Could you check a few things on this model? Use its own coordinates, in mm. Face numbers are marked on the shaded views. A direction names the side the tool comes from. Give positions to 0.01 mm unless a question says otherwise; leave off trailing zeros. Write each loop counter-clockwise with the first axis right and the second up, starting at its lowest first coordinate (ties: lowest second). Pieces come first, ordered by that corner, then holes. Notation, with made-up numbers: (69, 72) - (76, 72) arc R18 ccw to (76, 82) - close; hole circle Ø7 at (10.5, 21). An arc over 180 degrees is marked (long way). Write item = value, one per line.
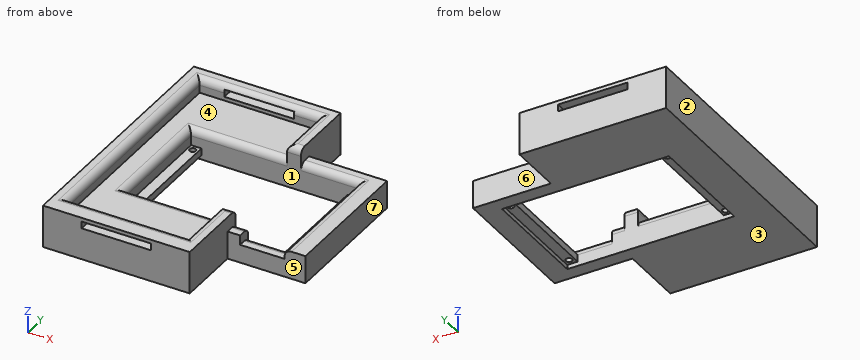
from build123d import *

# Parameters (mm, degrees)
F0_W      = 76.2
F0_H      = 50.8
F1_DEPTH  = 20.32
F2_W      = 60.96
F2_H      = 40.64
F3_DEPTH  = 17.272
F5_W      = 3.81
F5_H      = 40.64
F5_R      = 1.13665
F6_DEPTH  = 2.54
F8_W      = 16.256
F8_H      = 5.08
F9_DEPTH  = 3.4925
F11_DEPTH = 5.334
F13_DEPTH = 20.32
F14_R     = 2.54
F15_W     = 93.98
F15_H     = 10.16
F16_DEPTH = 82.042
F17_W     = 25.4
F17_H     = 2.54
F18_DEPTH = 93.98


with BuildPart() as f1:
    # F0 (on Top) → F1 (new body)
    with BuildSketch(Plane.XY):
        Rectangle(F0_W, F0_H)
    extrude(amount=F1_DEPTH)

    # F2 (on face) → F3 (cut)
    with BuildSketch(Plane.XY.offset(20.32)):
        Rectangle(F2_W, F2_H)
    extrude(amount=-F3_DEPTH, mode=Mode.SUBTRACT)

    # F5 (on offset) → F6 (join)
    with BuildSketch(Plane.XY.offset(11.7475)):
        with Locations((-28.575, 0)):
            Rectangle(F5_W, F5_H)
        with Locations((-28.575, -18.1356)):
            Circle(F5_R, mode=Mode.SUBTRACT)
        with Locations((-28.575, 18.1356)):
            Circle(F5_R, mode=Mode.SUBTRACT)
        with Locations((28.575, 0)):
            Rectangle(F5_W, F5_H)
        with Locations((28.575, -18.1356)):
            Circle(F5_R, mode=Mode.SUBTRACT)
        with Locations((28.575, 18.1356)):
            Circle(F5_R, mode=Mode.SUBTRACT)
    extrude(amount=F6_DEPTH)

    # F8 (on offset) → F9 (cut, through all)
    with BuildSketch(Plane.XY.offset(16.8275)):
        with Locations((22.352, -22.86)):
            Rectangle(F8_W, F8_H)
    extrude(amount=F9_DEPTH, mode=Mode.SUBTRACT)

    # F10 (on face) → F11 (join)
    with BuildSketch(Plane.XY.offset(20.32)):
        Polygon((-38.862, -41.3258), (-38.862, 39.9542), (4.572, 39.9542), (4.572, 20.32), (9.652, 20.32), (9.652, 45.0342), (-43.942, 45.0342), (-43.942, -48.9458), (9.652, -48.9458), (9.652, -20.32), (4.572, -20.32), (4.572, -41.3258), align=None)
    extrude(amount=F11_DEPTH)

    # F12 (on face) → F13 (join, through all)
    with BuildSketch(Plane(origin=(0, 0, 0), x_dir=(1, 0, 0), z_dir=(0, 0, -1))):
        Polygon((-43.942, 48.9458), (-43.942, -45.0342), (9.652, -45.0342), (9.652, -25.4), (-38.1, -25.4), (-38.1, 25.4), (9.652, 25.4), (9.652, 48.9458), align=None)
    extrude(amount=-F13_DEPTH)

    # F14
    f14_edges = [f1.edges().sort_by_distance(p)[0] for p in [
        (-12.954, 20.32, 20.32),
        (-30.48, 0, 20.32),
        (30.48, -2.54, 20.32),
        (-17.145, 39.9542, 25.654),
        (-38.862, -0.6858, 25.654),
        (-17.145, -41.3258, 25.654),
        (4.572, -30.8229, 25.654),
        (4.572, 30.1371, 25.654),
        (22.352, -20.32, 16.8275),
        (11.938, -20.32, 20.32),
        (-12.954, -20.32, 20.32),
        (20.066, 20.32, 20.32),
        (7.112, 20.32, 25.654),
        (7.112, -20.32, 25.654),
    ]]
    fillet(f14_edges, radius=F14_R)

    # F15 (on face) → F16 (cut, through all)
    with BuildSketch(Plane.YZ.offset(38.1)):
        with Locations((-1.9558, 5.08)):
            Rectangle(F15_W, F15_H)
    extrude(amount=-F16_DEPTH, mode=Mode.SUBTRACT)

    # F17 (on face) → F18 (cut, through all)
    with BuildSketch(Plane.XZ.offset(48.9458)):
        with Locations((-17.145, 22.987)):
            Rectangle(F17_W, F17_H)
    extrude(amount=-F18_DEPTH, mode=Mode.SUBTRACT)


solid = f1.part
1. Thinking about a two-plate mould opening in X: for the marked faces 1, 2, 3 and 4, which applies, pulls with the +X half, pulls with the -X half, needs draft (parallel to the pull), parting line crosses it, or undercut?
Filled sheet:
face_1 = undercut
face_2 = pulls with the -X half
face_3 = needs draft
face_4 = undercut
2. If we section it at C-C, the plane y = -37: Please give me the cut outline in (x, z), and give its area (3 significant figures).
Filled sheet:
outline = (-43.94, 10.16) - (9.65, 10.16) - (9.65, 25.65) - (7.11, 25.65) arc R2.54 ccw to (4.57, 23.11) - (4.57, 20.32) - (-38.86, 20.32) - (-38.86, 23.11) arc R2.54 ccw to (-41.4, 25.65) - (-43.94, 25.65) - close
area = 596 mm2
3. I need wall thicknesses on line 1 (X direction, y = -25, z = 21.75); line 2 (Y direction, x = -14, z = 12.25); line 3 (Y direction, x = -12.5, z = 21). Which ranges of each line are inside material? Lowest first, please.
Filled sheet:
line_1 = -43.94 to -38.86, 4.57 to 9.65
line_2 = -48.95 to -20.32, 20.32 to 45.03
line_3 = -48.95 to -41.33, 39.95 to 45.03
4. For pin 1 (2.5 mm diameter, centred on x = 28.58, y = 18.14, fed in from -Z); pin 2 (12 mm diameter, centred on x = -3.5, y = -30, fed in from +Z); pin 3 (0.8 mm diameter, centred on x = -24.5, z = 22, fed in from +Y); pin 4 (8 mm diameter, centred on x = 24.5, z = 13.5, fed in from +Y), each with a flat end and sliding along its axis, tell me the tip position at first contact or that it passes through.
Filled sheet:
pin_1 = 11.75
pin_2 = 20.32
pin_3 = 45.03
pin_4 = 25.4
5. If we section it at D-D, the plane x = -28.5: Count the separate pieces of the cut face and the enclosed holes in it, and give its area (3 significant figures).
Filled sheet:
separate_pieces = 5
enclosed_holes = 0
area = 664 mm2
6. If we section it at B-B, the plane y = -8: Please give me the cut outline in (x, z), and give its area (3 significant figures).
Filled sheet:
outline = (-43.94, 10.16) - (-30.48, 10.16) - (-30.48, 11.75) - (-26.67, 11.75) - (-26.67, 14.29) - (-30.48, 14.29) - (-30.48, 17.78) arc R2.54 ccw to (-33.02, 20.32) - (-38.86, 20.32) - (-38.86, 23.11) arc R2.54 ccw to (-41.4, 25.65) - (-43.94, 25.65) - close; (26.67, 11.75) - (30.48, 11.75) - (30.48, 10.16) - (38.1, 10.16) - (38.1, 20.32) - (33.02, 20.32) arc R2.54 ccw to (30.48, 17.78) - (30.48, 14.29) - (26.67, 14.29) - close
area = 256 mm2
7. If we section it at A-A, the plane x = -11: Please give me the cut outline in (y, z).
Filled sheet:
outline = (-48.95, 10.16) - (-20.32, 10.16) - (-20.32, 17.78) arc R2.54 ccw to (-22.86, 20.32) - (-41.33, 20.32) - (-41.33, 21.72) - (-48.95, 21.72) - close; (-48.95, 24.26) - (-41.6, 24.26) arc R2.54 ccw to (-43.87, 25.65) - (-48.95, 25.65) - close; (20.32, 10.16) - (45.03, 10.16) - (45.03, 21.72) - (39.95, 21.72) - (39.95, 20.32) - (22.86, 20.32) arc R2.54 ccw to (20.32, 17.78) - close; (40.23, 24.26) - (45.03, 24.26) - (45.03, 25.65) - (42.49, 25.65) arc R2.54 ccw to start
8. Which directions (+Z, -Z, +X, -X, +Y, -Y) give clear straight access to the entire face, cutting with the end or side of a thin tool? Please do the marked faces 5, 6 and 7.
Filled sheet:
face_5 = +Z, -Z, +X, -Y
face_6 = +Z, -Z, +X, +Y
face_7 = +Z, -Z, +X, +Y, -Y
